Verification items for the finished model (mm, model axes). Round coordinates to 2 decimals unless told otherwise and drop trailing zeros. Order: outer loops, then holes, each group sorted by start corner. A loop starts at its lowest first (then second) coordinate and runs counter-clockwise, first axis right, second up. Notation, with made-up numbers: M -27,76.25 L -18,76.25 A19 ccw -18,107.25 Z; hole C 36.5,10 d1. An arc over 180 degrees is marked long. Answer as a JSON object with one key per item and string values. Group by question number.
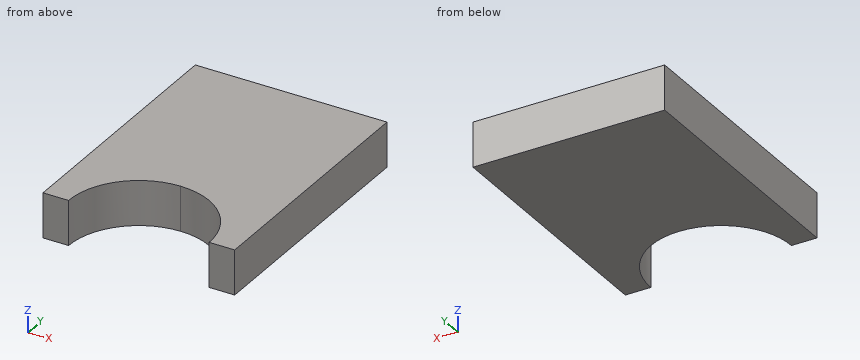
```python
from build123d import *

# Parameters (mm, degrees)
F1_DEPTH = 7


with BuildPart() as f1:
    # F0 (on Top) → F1 (new body)
    with BuildSketch(Plane.XY):
        with BuildLine():
            ThreePointArc((-11, 0), (-7.778175, 7.778175), (0, 11))
            Line((0, 11), (0, 40))
            Line((0, 40), (-15, 40))
            Line((-15, 40), (-15, 0))
            Line((-15, 0), (-11, 0))
        make_face()
        with BuildLine():
            ThreePointArc((0, 11), (7.778175, 7.778175), (11, 0))
            Line((11, 0), (15, 0))
            Line((15, 0), (15, 40))
            Line((15, 40), (0, 40))
            Line((0, 40), (0, 11))
        make_face()
    extrude(amount=F1_DEPTH)


solid = f1.part
```
Q1. Cross-section at B-B, the plane z = 1.5. Record the cut outline in (x, y), then the cut area to 3 significant figures.
Q2. Cross-section at A-A, the plane y = 10.5. Record the cut outline in (x, z), then the cut area to 3 significant figures.
Q3. Thickness scan on line 1 (X direction, y = 5, z = 4.5); line 2 (X direction, y = 9, z = 3.25); line 3 (Y direction, x = 1.5, z = 4.5). Record the ranges inside material, lowest first. Write a range as from..to.
Q4. Gauge pin test, flat end, axial feed: pin 1 Ø4 at (x, y) = (1, 8) entering from +Z. Record the tip position at first contact, or that the pin passes through.
Q5. Cross-section at D-D, the plane x = -0.5. Record the cut outline in (y, z), then the cut area to 3 significant figures.
Q6. Cross-section at C-C, the plane x = 3.75. Record the cut outline in (y, z), then the cut area to 3 significant figures.
Conclusion:
{
 "1": {"outline": "M -15,0 L -11,0 A11 cw 0,11 A11 cw 11,0 L 15,0 L 15,40 L -15,40 Z", "area": "1,010 mm2"},
 "2": {"outline": "M -15,0 L -3.28,0 L -3.28,7 L -15,7 Z; M 3.28,0 L 15,0 L 15,7 L 3.28,7 Z", "area": "164 mm2"},
 "3": {"line 1": "-15..-9.8, 9.8..15", "line 2": "-15..-6.32, 6.32..15", "line 3": "10.9..40"},
 "4": {"pin 1": "through"},
 "5": {"outline": "M 10.99,0 L 40,0 L 40,7 L 10.99,7 Z", "area": "203 mm2"},
 "6": {"outline": "M 10.34,0 L 40,0 L 40,7 L 10.34,7 Z", "area": "208 mm2"}
}
